Design review of the part built by this model. Coordinates are the model's own, in mm. A direction names the side the tool comes from. Give positions to 0.01 mm unless a question says otherwise; leave off trailing zeros. Write each loop counter-clockwise with the first axis right and the second up, starting at its lowest first coordinate (ties: lowest second). Pieces come first, ordered by that corner, then holes. Notation, with made-up numbers: (-0.75, 22) -> (41.25, 22) arc R11 cw to (41.25, 35) -> close; hole circle Ø6 at (-34, 26.5). An arc over 180 degrees is marked (long way). Answer as a JSON object with one key per item and string values.
```python
from build123d import *

# Parameters (mm, degrees)
F1_DEPTH = 25.4
F3_DEPTH = 6.35
F5_DEPTH = 19.05
F6_R     = 6.35
F7_DEPTH = 25.4010001
F8_R     = 3.175
F9_DEPTH = 6.3510001


with BuildPart() as f1:
    # F0 (on Front) → F1 (new body)
    with BuildSketch(Plane.XZ):
        with BuildLine():
            add(Edge.make_bspline(
                [(-43.2595827852, 47.5290406017), (-40.4437585235, 36.3493184584), (-37.6279342618, 25.1695963151), (-25.0532810608, 24.9273501791)],
                knots=[0, 0, 0, 0, 0.3387649469, 0.3387649469, 0.3387649469, 0.3387649469], degree=3))
            Line((-43.2595827852, 47.5290406017), (-43.2595827852, 24.9273501791))
            Line((-43.2595827852, 24.9273501791), (-25.0532810608, 24.9273501791))
        make_face()
        with BuildLine():
            Line((-24.2095827852, 24.9273501791), (-25.0532810608, 24.9273501791))
            add(Edge.make_bspline(
                [(-25.0532810608, 24.9273501791), (-24.776800624, 24.9220238837), (-24.495602442, 24.9219851311), (-24.2095827852, 24.9273501791)],
                knots=[0.3387649469, 0.3387649469, 0.3387649469, 0.3387649469, 0.3462134132, 0.3462134132, 0.3462134132, 0.3462134132], degree=3))
        make_face()
        with BuildLine():
            add(Edge.make_bspline(
                [(-72.6796290961, 24.9273501791), (-73.3463645358, 24.7120564737), (-74.1177900306, 24.7018207484), (-75.0095827852, 24.9273501791)],
                knots=[0.2357769442, 0.2357769442, 0.2357769442, 0.2357769442, 0.2710842466, 0.2710842466, 0.2710842466, 0.2710842466], degree=3))
            Line((-72.6796290961, 24.9273501791), (-75.0095827852, 24.9273501791))
        make_face()
        with BuildLine():
            Line((-68.6595827852, 24.9273501791), (-68.6595827852, 36.1707942024))
            add(Edge.make_bspline(
                [(-68.6595827852, 36.1707942024), (-68.9307748645, 30.329459196), (-69.8866500944, 25.8292233399), (-72.6796290961, 24.9273501791)],
                knots=[0.0878733709, 0.0878733709, 0.0878733709, 0.0878733709, 0.2357769442, 0.2357769442, 0.2357769442, 0.2357769442], degree=3))
            Line((-72.6796290961, 24.9273501791), (-68.6595827852, 24.9273501791))
        make_face()
        with BuildLine():
            ThreePointArc((-68.6490277589, 47.0113667108), (-68.6569437544, 47.2701498593), (-68.6595827852, 47.5290406017))
            Line((-68.6595827852, 47.5290406017), (-68.6595827852, 36.1707942024))
            add(Edge.make_bspline(
                [(-68.6490277589, 47.0113667108), (-68.5724341976, 43.2409261553), (-68.5055106798, 39.4894264591), (-68.6595827852, 36.1707942024)],
                knots=[0.0038450504, 0.0038450504, 0.0038450504, 0.0038450504, 0.0878733709, 0.0878733709, 0.0878733709, 0.0878733709], degree=3))
        make_face()
        with BuildLine():
            add(Edge.make_bspline(
                [(-68.6595827852, 47.5290406017), (-68.6560576938, 47.356469418), (-68.6525326024, 47.1838982344), (-68.6490277589, 47.0113667108)],
                knots=[0, 0, 0, 0, 0.0038450504, 0.0038450504, 0.0038450504, 0.0038450504], degree=3))
            ThreePointArc((-68.6595827852, 47.5290406017), (-68.6569437544, 47.2701498593), (-68.6490277589, 47.0113667108))
        make_face()
        with BuildLine():
            Line((-43.2595827852, 24.9273501791), (-43.2595827852, 47.5290406017))
            ThreePointArc((-43.2595827852, 47.5290406017), (-55.7006920428, 34.8316796324), (-68.6490277589, 47.0113667108))
            add(Edge.make_bspline(
                [(-68.6490277589, 47.0113667108), (-68.5724341976, 43.2409261553), (-68.5055106798, 39.4894264591), (-68.6595827852, 36.1707942024)],
                knots=[0.0038450504, 0.0038450504, 0.0038450504, 0.0038450504, 0.0878733709, 0.0878733709, 0.0878733709, 0.0878733709], degree=3))
            Line((-68.6595827852, 36.1707942024), (-68.6595827852, 24.9273501791))
            Line((-68.6595827852, 24.9273501791), (-72.6796290961, 24.9273501791))
            add(Edge.make_bspline(
                [(-72.6796290961, 24.9273501791), (-73.3463645358, 24.7120564737), (-74.1177900306, 24.7018207484), (-75.0095827852, 24.9273501791)],
                knots=[0.2357769442, 0.2357769442, 0.2357769442, 0.2357769442, 0.2710842466, 0.2710842466, 0.2710842466, 0.2710842466], degree=3))
            Line((-75.0095827852, 24.9273501791), (-75.0095827852, 18.5773501791))
            Line((-75.0095827852, 18.5773501791), (-24.2095827852, 18.5773501791))
            Line((-24.2095827852, 18.5773501791), (-24.2095827852, 24.9273501791))
            add(Edge.make_bspline(
                [(-25.0532810608, 24.9273501791), (-24.776800624, 24.9220238837), (-24.495602442, 24.9219851311), (-24.2095827852, 24.9273501791)],
                knots=[0.3387649469, 0.3387649469, 0.3387649469, 0.3387649469, 0.3462134132, 0.3462134132, 0.3462134132, 0.3462134132], degree=3))
            Line((-25.0532810608, 24.9273501791), (-43.2595827852, 24.9273501791))
        make_face()
        with BuildLine():
            ThreePointArc((-43.2595827852, 47.5290406017), (-46.9793266641, 56.5092967228), (-55.9595827852, 60.2290406017))
            ThreePointArc((-55.9595827852, 60.2290406017), (-64.9398389062, 56.5092967228), (-68.6595827852, 47.5290406017))
            add(Edge.make_bspline(
                [(-68.6595827852, 47.5290406017), (-68.6560576938, 47.356469418), (-68.6525326024, 47.1838982344), (-68.6490277589, 47.0113667108)],
                knots=[0, 0, 0, 0, 0.0038450504, 0.0038450504, 0.0038450504, 0.0038450504], degree=3))
            ThreePointArc((-68.6490277589, 47.0113667108), (-55.7006920428, 34.8316796324), (-43.2595827852, 47.5290406017))
        make_face()
    extrude(amount=F1_DEPTH)

    # F2 (on face) → F3 (join)
    with BuildSketch(Plane.XZ.offset(25.4)):
        with BuildLine():
            add(Edge.make_bspline(
                [(-43.2595827852, 47.5290406017), (-40.4437585235, 36.3493184584), (-37.6279342618, 25.1695963151), (-25.0532810608, 24.9273501791)],
                knots=[0, 0, 0, 0, 0.3387649469, 0.3387649469, 0.3387649469, 0.3387649469], degree=3))
            ThreePointArc((-43.2595827852, 47.5290406017), (-55.9595827852, 34.8290406017), (-68.6595827852, 47.5290406017))
            Line((-68.6595827852, 47.5290406017), (-68.6595827852, 36.1707942024))
            add(Edge.make_bspline(
                [(-68.6595827852, 36.1707942024), (-68.9307748645, 30.329459196), (-69.8866500944, 25.8292233399), (-72.6796290961, 24.9273501791)],
                knots=[0.0878733709, 0.0878733709, 0.0878733709, 0.0878733709, 0.2357769442, 0.2357769442, 0.2357769442, 0.2357769442], degree=3))
            Line((-72.6796290961, 24.9273501791), (-75.0095827852, 24.9273501791))
            Line((-75.0095827852, 24.9273501791), (-75.0095827852, 18.5773501791))
            Line((-75.0095827852, 18.5773501791), (-24.2095827852, 18.5773501791))
            Line((-24.2095827852, 18.5773501791), (-24.2095827852, 24.9273501791))
            Line((-24.2095827852, 24.9273501791), (-25.0532810608, 24.9273501791))
        make_face()
    extrude(amount=F3_DEPTH)

    # F4 (on face) → F5 (cut)
    with BuildSketch(Plane.XZ.offset(31.75)):
        with BuildLine():
            add(Edge.make_bspline(
                [(-68.6595827852, 36.1707942024), (-68.9307748645, 30.329459196), (-69.8866500944, 25.8292233399), (-72.6796290961, 24.9273501791)],
                knots=[0.0878733709, 0.0878733709, 0.0878733709, 0.0878733709, 0.2357769442, 0.2357769442, 0.2357769442, 0.2357769442], degree=3))
            Line((-72.6796290961, 24.9273501791), (-25.0532810608, 24.9273501791))
            add(Edge.make_bspline(
                [(-43.2595827852, 47.5290406017), (-40.4437585235, 36.3493184584), (-37.6279342618, 25.1695963151), (-25.0532810608, 24.9273501791)],
                knots=[0, 0, 0, 0, 0.3387649469, 0.3387649469, 0.3387649469, 0.3387649469], degree=3))
            ThreePointArc((-43.2595827852, 47.5290406017), (-55.9595827852, 34.8290406017), (-68.6595827852, 47.5290406017))
            Line((-68.6595827852, 47.5290406017), (-68.6595827852, 36.1707942024))
        make_face()
    extrude(amount=-F5_DEPTH, mode=Mode.SUBTRACT)

    # F6 (on face) → F7 (cut, through all)
    with BuildSketch(Plane.XZ.offset(25.4)):
        with Locations((-55.9595827852, 47.5290406017)):
            Circle(F6_R)
    extrude(amount=-F7_DEPTH, mode=Mode.SUBTRACT)

    # F8 (on face) → F9 (cut, through all)
    with BuildSketch(Plane.XY.offset(24.9273501791)):
        with Locations((-65.4845827852, -22.225)):
            Circle(F8_R)
        with Locations((-33.7345827852, -22.225)):
            Circle(F8_R)
    extrude(amount=-F9_DEPTH, mode=Mode.SUBTRACT)


solid = f1.part
```
(1) We need section A-A, the plane y = -20. State the section outline as (x, z) points.
Here are the results:
{"outline": "(-75.01, 18.58) -> (-67.75, 18.58) -> (-67.75, 24.93) -> (-75.01, 24.93) -> close; circle Ø25.4 at (-55.96, 47.53); (-63.22, 18.58) -> (-36, 18.58) -> (-36, 24.93) -> (-63.22, 24.93) -> close; (-31.47, 18.58) -> (-24.21, 18.58) -> (-24.21, 24.93) -> (-31.47, 24.93) -> close; hole circle Ø12.7 at (-55.96, 47.53)"}
(2) We need section C-C, the plane x = -64. State the section outline as (y, z) points, then the cut area to 3 significant figures.
Here are the results:
{"outline": "(-31.75, 18.58) -> (-25.03, 18.58) -> (-25.03, 24.93) -> (-31.75, 24.93) -> close; (-25.4, 37.7) -> (-12.7, 37.7) -> (-12.7, 24.93) -> (-19.42, 24.93) -> (-19.42, 18.58) -> (0, 18.58) -> (0, 57.36) -> (-25.4, 57.36) -> close", "area": "828 mm²"}
(3) For line 1 along Y through (x, z) = (-60.5, 43); line 2 along Y through (x, z) = (-43, 46); line 3 along Y through (x, z) = (-63.5, 24), list the stretches that pass through material, from the lowest coordinate up.
Here are the results:
{"line 1": "y = -25.4 to 0", "line 2": "y = -12.7 to 0", "line 3": "y = -31.75 to -24.7, -19.75 to 0"}
(4) Clearance check with flat-ended pins moving along their axes: pin 1 (9.5 mm diameter, centred on x = -41, y = -14, fed in from +Z); pin 2 (12.5 mm diameter, centred on y = -4, z = 42.5, fed in from -X); pin 3 (12.5 mm diameter, centred on x = -62, z = 49.5, fed in from -Y). State where each tip first meets the part, or that it passes through.
Here are the results:
{"pin 1": "stops at z = 55.08", "pin 2": "stops at x = -68.66", "pin 3": "stops at y = -25.4"}
(5) For faces 4 (the cylindrical face through (-52.546, -12.878, 52.883)), 5 (the cylindrical face through (-62.456, -21.271, 21.797)), 6 (the flat face through (-50, -25.4, 51)), list the 3-axis set-ups (+Z, -Z, +X, -X, +Y, -Y) from which the entire face can be reached by the end or side of a thin tool; tool diameter is ignored.
Here are the results:
{"face 4": "+Y, -Y", "face 5": "-Z", "face 6": "+Z, +X, -X, -Y"}
(6) We need section D-D, the plane y = -23.5. State the section outline as (x, z) points, then the cut area to 3 significant figures.
Here are the results:
{"outline": "(-75.01, 18.58) -> (-68.39, 18.58) -> (-68.39, 24.93) -> (-75.01, 24.93) -> close; circle Ø25.4 at (-55.96, 47.53); (-62.58, 18.58) -> (-36.64, 18.58) -> (-36.64, 24.93) -> (-62.58, 24.93) -> close; (-30.83, 18.58) -> (-24.21, 18.58) -> (-24.21, 24.93) -> (-30.83, 24.93) -> close; hole circle Ø12.7 at (-55.96, 47.53)", "area": "629 mm²"}
(7) We need section B-B, the plane y = -15. State the section outline as (x, z) points, then the cut area to 3 significant figures.
Here are the results:
{"outline": "(-75.01, 18.58) -> (-24.21, 18.58) -> (-24.21, 24.93) -> (-75.01, 24.93) -> close; circle Ø25.4 at (-55.96, 47.53); hole circle Ø12.7 at (-55.96, 47.53)", "area": "703 mm²"}
(8) The part is to be moulded in two halves that separate along Z. For faces 1 (the flat face through (-49, -12.7, 31)), 2 (the flat face through (-50, -16, 18.577)), 3 (the flat face through (-68.66, -6, 42)), say which applies: +Z half, -Z half, draft (parallel to the pull), parting line (faces both ways), or undercut.
Here are the results:
{"face 1": "undercut", "face 2": "-Z half", "face 3": "draft"}
